Could you check a few things on this model? Use its own coordinates, in mm. Give positions to 0.01 mm unless a question says otherwise; leave off trailing zeros. Write each loop counter-clockwise with the first axis right and the second up, starting at its lowest first coordinate (ties: lowest second). Pieces come first, ordered by that corner, then holes. Notation, with made-up numbers: (0, 30) - (7, 30) arc R22 cw to (7, 48) - close; hole circle Ø3 at (-35, -9). An arc over 180 degrees is marked (long way). Answer in a Markdown table with one row per item.
Autodesk Fusion 360 part; units mm, degrees
sketch "Sketch1" plane through (0, 0, 0) normal (0, 0, 1) x (1, 0, 0)
  line L0 (-5.7735, 10) -> (-11.547, 0)
  line L1 (-11.547, 0) -> (-5.7735, -10)
  line L2 (-5.7735, -10) -> (5.7735, -10)
  line L3 (5.7735, -10) -> (11.547, 0)
  line L4 (11.547, 0) -> (5.7735, 10)
  line L5 (5.7735, 10) -> (-5.7735, 10)
  circle A0 centre (0, 0) radius 1.625
  circle A1 centre (-3.25, 5.6292) radius 2.05
  line L6 (0, 0) -> (-5.7735, 10) construction
  circle A2 centre (-6.5, 0) radius 2.05
  circle A3 centre (-3.25, -5.6292) radius 2.05
  circle A4 centre (3.25, -5.6292) radius 2.05
  circle A5 centre (6.5, 0) radius 2.05
  circle A6 centre (3.25, 5.6292) radius 2.05
  circle A7 centre (0, 0) radius 6.5 construction
  dimension "d1" = 10
  dimension "d2" = 3.25
  dimension "d4" = 4.1
  dimension "d9" = 360
  dimension "d10" = 13
extrude "Extrude1" add sketch "Sketch1" along normal blind 8
chamfer "Chamfer2" distance 0.3 angle 45 7 edges at (-8.4113, 0.7413, 8) (-5.1613, 6.3705, 8) (-1.515, 0.5876, 8) (-5.1613, -4.8879, 8) (1.3387, -4.8879, 8) (4.5887, 0.7413, 8) (1.3387, 6.3705, 8)
chamfer "Chamfer3" distance 0.5 angle 45 1 edges at (-1.515, 0.5876, 0)
fillet "Fillet1" radius 0.5 6 edges at (-5.7735, -10, 4) (5.7735, -10, 4) (11.547, 0, 4) (5.7735, 10, 4) (-5.7735, 10, 4) (-11.547, 0, 4)
chamfer "Chamfer4" distance 0.3 angle 45 12 edges at (0, -10, 8) (5.7348, -9.933, 8) (8.6603, -5, 8) (11.4697, 0, 8) (8.6603, 5, 8) (5.7348, 9.933, 8) (0, 10, 8) (-5.7348, 9.933, 8) (-8.6603, 5, 8) (-11.4697, 0, 8) (-8.6603, -5, 8) (-5.7348, -9.933, 8)
1) Will these pins go through, and if not, where does the flat tip stop? P1, Ø1, axis at y = -8, z = 6.5, coming from the -X side; P2, Ø3, axis at x = -8.5, z = 5, coming from the +Y side; P3, Ø1, axis at x = 0.5, y = -0.5, coming from the -Z side (3 decimals).
Check values:
| item | result |
|---|---|
| P1 | stops at x = -7.22 |
| P2 | stops at y = 7.88 |
| P3 | passes through |
2) Imagine slicing it at C-C (x = 6.5). List the corners of the cut face in (y, z) for me, then the cut area to 3 significant figures.
Check values:
| item | result |
|---|---|
| outline | (-8.74, 0) - (-2.05, 0) - (-2.05, 7.7) - (-2.35, 8) - (-8.14, 8) - (-8.74, 7.7) - close; (2.05, 0) - (8.74, 0) - (8.74, 7.7) - (8.14, 8) - (2.35, 8) - (2.05, 7.7) - close |
| area | 107 mm2 |
3) If I drill on line 1 (Y direction, x = -3.25, z = 5); line 2 (Y direction, x = 0, z = 4) (3 decimals); line 3 (X direction, y = -4.75, z = 1.5), over which ranges is the centre line in solid material (lowest first)?
Check values:
| item | result |
|---|---|
| line 1 | y = -10 to -7.68, -3.58 to 3.58, 7.68 to 10 |
| line 2 | y = -10 to -1.625, 1.625 to 10 |
| line 3 | x = -8.8 to -5.1, -1.4 to 1.4, 5.1 to 8.8 |
4) Imagine slicing it at A-A (x = 3.25). List the corners of the cut face in (y, z) for me.
Check values:
| item | result |
|---|---|
| outline | (-10, 0) - (-7.68, 0) - (-7.68, 7.7) - (-7.98, 8) - (-9.7, 8) - (-10, 7.7) - close; (-3.58, 0) - (3.58, 0) - (3.58, 7.7) - (3.28, 8) - (-3.28, 8) - (-3.58, 7.7) - close; (7.68, 0) - (10, 0) - (10, 7.7) - (9.7, 8) - (7.98, 8) - (7.68, 7.7) - close |
5) Imagine slicing it at D-D (y = -3). List the corners of the cut face in (x, z) for me, then the cut area to 3 significant figures.
Check values:
| item | result |
|---|---|
| outline | (-9.81, 0) - (9.81, 0) - (9.81, 7.7) - (9.47, 8) - (-9.47, 8) - (-9.81, 7.7) - close |
| area | 157 mm2 |
6) Imagine slicing it at B-B (z = 1.25). List the corners of the cut face in (x, y) for me (3 decimals), then the cut area to 3 significant figures.
Check values:
| item | result |
|---|---|
| outline | (-11.403, -0.25) - (-5.918, -9.75) arc R0.5 ccw to (-5.485, -10) - (5.485, -10) arc R0.5 ccw to (5.918, -9.75) - (11.403, -0.25) arc R0.5 ccw to (11.403, 0.25) - (5.918, 9.75) arc R0.5 ccw to (5.485, 10) - (-5.485, 10) arc R0.5 ccw to (-5.918, 9.75) - (-11.403, 0.25) arc R0.5 ccw to start; hole circle Ø4.1 at (-6.5, 0); hole circle Ø4.1 at (-3.25, -5.629); hole circle Ø4.1 at (-3.25, 5.629); hole circle Ø3.25 at (0, 0); hole circle Ø4.1 at (3.25, -5.629); hole circle Ø4.1 at (3.25, 5.629); hole circle Ø4.1 at (6.5, 0) |
| area | 259 mm2 |
